```python
from build123d import *

# Parameters (mm, degrees)
F0_W     = 86.5
F0_H     = 370
F1_DEPTH = 10
F3_DEPTH = 4
F4_W     = 12
F4_H     = 370
F5_DEPTH = 6


with BuildPart() as f1:
    # F0 (on Front) → F1 (new body)
    with BuildSketch(Plane.XZ):
        Rectangle(F0_W, F0_H)
    extrude(amount=F1_DEPTH)

    # F2 (on face) → F3 (cut)
    with BuildSketch(Plane.XZ.offset(10)):
        Polygon((-43.25, 185), (-43.25, 173), (31.25, 173), (31.25, -173), (-43.25, -173), (-43.25, -185), (43.25, -185), (43.25, 185), align=None)
    extrude(amount=-F3_DEPTH, mode=Mode.SUBTRACT)

    # F4 (on face) → F5 (cut)
    with BuildSketch(Plane(origin=(0, 0, 0), x_dir=(-1, 0, 0), z_dir=(0, 1, 0))):
        with Locations((37.25, 0)):
            Rectangle(F4_W, F4_H)
    extrude(amount=-F5_DEPTH, mode=Mode.SUBTRACT)


solid = f1.part
```
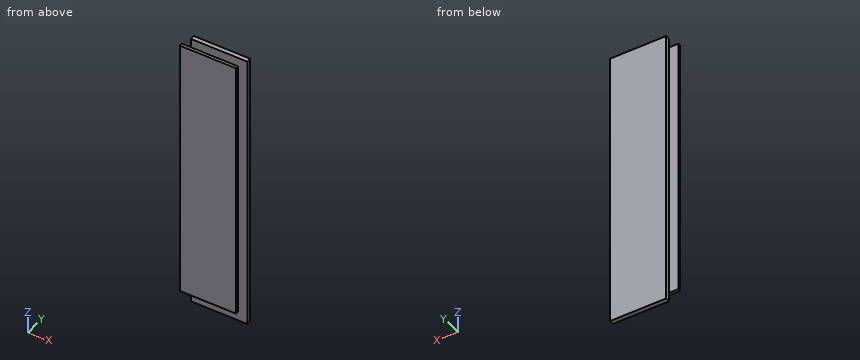
Design review of the part built by this model. Coordinates are the model's own, in mm. Give positions to 0.01 mm unless a question says otherwise; leave off trailing zeros. Write each loop counter-clockwise with the first axis right and the second up, starting at its lowest first coordinate (ties: lowest second). Pieces come first, ordered by that corner, then holes.
(1) Clearance check with flat-ended pins moving along their axes: pin 1 Ø9.5 at (x, z) = (-36.5, -61) entering from +Y; pin 2 Ø5 at (y, z) = (-2.5, 37) entering from -X; pin 3 Ø2 at (y, z) = (-8.5, -34.5) entering from +X; pin 4 Ø2 at (x, z) = (16.5, 53.5) entering from +Y. State where each tip first meets the part, or that it passes through.
Checked values:
pin 1: stops at y = -6
pin 2: stops at x = -31.25
pin 3: stops at x = 31.25
pin 4: stops at y = 0
(2) Add section A-A (z = -16). Give the boundary of the cut face in (x, y).
Checked values:
outline: (-43.25, -10) - (31.25, -10) - (31.25, -6) - (43.25, -6) - (43.25, 0) - (-31.25, 0) - (-31.25, -6) - (-43.25, -6) - close
(3) Add section B-B (x = 6.5). Give the boundary of the cut face in (y, z).
Checked values:
outline: (-10, -173) - (-6, -173) - (-6, -185) - (0, -185) - (0, 185) - (-6, 185) - (-6, 173) - (-10, 173) - close
(4) Wall thickness on line 1 along X through (y, z) = (-2.25, -109); line 2 along Y through (x, z) = (-32.5, -63); line 3 along X through (y, z) = (-6.5, -82): over which ranges is each line inside the solid? List them lowest first.
Checked values:
line 1: x = -31.25 to 43.25
line 2: y = -10 to -6
line 3: x = -43.25 to 31.25
(5) Add section C-C (y = -2.5). Give the boundary of the cut face in (x, z).
Checked values:
outline: (-31.25, -185) - (43.25, -185) - (43.25, 185) - (-31.25, 185) - close
